Geometry check sheet. Reference: the model listing, model coordinates, mm. Face numbers are marked on the shaded views. A direction names the side the tool comes from. Give positions to 0.01 mm unless a question says otherwise; leave off trailing zeros. Loops run counter-clockwise (first coordinate to the right, second up) from the corner with the lowest first, then second, coordinate; pieces in that order, holes last. Notation, with made-up numbers: (1.5, 29) - (53.5, 29) arc R22 ccw to (53.5, 55) - close; hole circle Ø10 at (72, 31.5). An arc over 180 degrees is marked (long way). One line per question, with ' | ' between items. Start each with the question number.
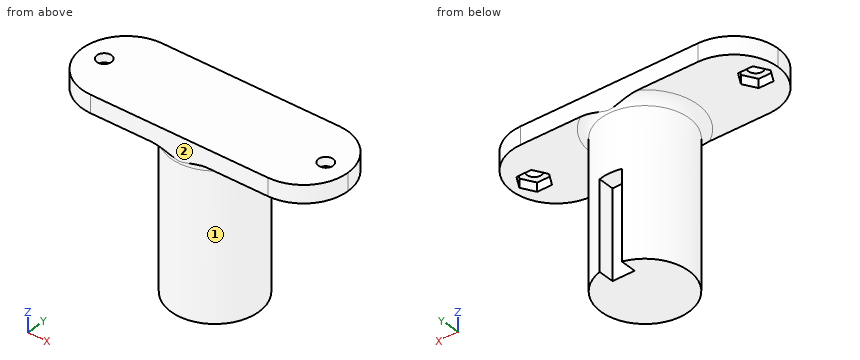
Autodesk Inventor part; units mm, degrees
ref_plane "YZ Plane" through (0, 0, 0) normal (1, 0, 0) x (0, 1, 0)
ref_plane "XZ Plane" through (0, 0, 0) normal (0, 1, 0) x (-1, 0, 0)
ref_plane "XY Plane" through (0, 0, 0) normal (0, 0, 1) x (1, 0, 0)
sketch "Sketch1" plane through (0, 0, 0) normal (0, 0, 1) x (1, 0, 0)
  line L0 (-30, -10) -> (30, -10)
  line L1 (30, -10) -> (30, 10)
  line L2 (30, 10) -> (-30, 10)
  line L3 (-30, 10) -> (-30, -10)
  line L4 (-30, -10) -> (30, 10) construction
  line L5 (30, -10) -> (-30, 10) construction
  circle A0 centre (0, 0) radius 9.9
  circle A1 centre (-25, 0) radius 1.65
  circle A2 centre (25, 0) radius 1.65
  line L6 (-25, 0) -> (25, 0) construction
  point P0 (-30, 0)
  dimension "d0" = 60
  dimension "d1" = 19.8
  dimension "d2" = 20
  dimension "d3" = 50
  dimension "d4" = 3.3
extrude "Extrusion1" add sketch "Sketch1" along normal blind 4 contours L3 L2 L1 L0 | A0
extrude "Extrusion2" add sketch "Sketch1" against normal blind 35 contours A0
fillet "Fillet1" radius 2 1 edges at (-9.9, 0, 0)
fillet "Fillet2" radius 10 4 edges at (30, 10, 2) (30, -10, 2) (-30, 10, 2) (-30, -10, 2)
sketch "Sketch2" plane through (0, 0, -35) normal (0, 0, -1) x (-1, 0, 0)
  circle A0 centre (0, 0) radius 9.9
  line L0 (-2.5, 0) -> (2.5, 0)
  line L1 (2.5, 0) -> (2.5, 12)
  line L2 (2.5, 12) -> (-2.5, 12)
  line L3 (-2.5, 12) -> (-2.5, 0)
  line L4 (-2.5, 6) -> (2.5, 6)
  point P0 (0, 12)
  point P1 (2.5, 9.5791)
  point P2 (-2.5, 9.5791)
  dimension "d11" = 12
  dimension "d12" = 5
  dimension "d13" = 6
extrude "Extrusion3" cut sketch "Sketch2" against normal blind 20 contours L1 L4 L3 A0
sketch "Sketch3" plane through (0, 0, 0) normal (0, 0, -1) x (-1, 0, 0)
  arc A0 (-20, 10) -> (-20, -10) centre (-20, 0) ccw
  line L0 (-6.4506, -10) -> (-20, -10)
  arc A1 (-6.4506, 10) -> (-6.4506, -10) centre (0, 0) ccw
  line L1 (-20, 10) -> (-6.4506, 10)
  circle A2 centre (-25, 0) radius 1.65
  line L2 (-28.3486, 0) -> (-26.6743, 2.9)
  line L3 (-26.6743, 2.9) -> (-23.3257, 2.9)
  line L4 (-23.3257, 2.9) -> (-21.6514, 0)
  line L5 (-21.6514, 0) -> (-23.3257, -2.9)
  line L6 (-23.3257, -2.9) -> (-26.6743, -2.9)
  line L7 (-26.6743, -2.9) -> (-28.3486, 0)
  circle A3 centre (25, 0) radius 1.65
  line L8 (23.3257, 2.9) -> (26.6743, 2.9)
  line L9 (26.6743, 2.9) -> (28.3486, 0)
  line L10 (28.3486, 0) -> (26.6743, -2.9)
  line L11 (26.6743, -2.9) -> (23.3257, -2.9)
  line L12 (23.3257, -2.9) -> (21.6514, 0)
  line L13 (21.6514, 0) -> (23.3257, 2.9)
  point P0 (-25, 2.9)
  dimension "d16" = 5.8
  dimension "d17" = 5.8
extrude "Extrusion4" cut sketch "Sketch3" against normal blind 2 contours L2 L3 L4 L5 L6 L7 | L8 L9 L10 L11 L12 L13
properties part number "GIRO_1" material "Steel, Mild, Welded"
(1) Tool access check on the marked faces 1 and 2. Record the directions out of +Z, -Z, +X, -X, +Y, -Y that give a thin tool (end or side, any length) a straight path to the whole face; none if there is none.
(2) Material ranges on line 1 (X direction, y = 0, z = 3); line 2 (Z direction, x = 10.5, y = 5.25); line 3 (Z direction, x = 22.5, y = 1.25), recorded low to high.
(3) Depth check by flat-ended pin: pin 1 Ø1.7 at (x, y) = (-24.5, -1) entering from -Z; pin 2 Ø1 at (x, z) = (25, 1.5) entering from -Y; pin 3 Ø3 at (y, z) = (0, -11) entering from -X. Enter the tip coordinate at first touch or a pass-through.
(4) Section check B-B, the plane x = 0. Record the boundary of the cut face in (y, z).
(5) Section check D-D, the plane x = 15.5. Record the boundary of the cut face in (y, z).
(6) Section check A-A, the plane x = 24. Record the boundary of the cut face in (y, z).
(7) Section check C-C, the plane z = -19.5. Record the boundary of the cut face in (x, y).
Numbers:
1) face 1: -Z | face 2: +Z, -Z, +X, -X, -Y
2) line 1: -30 to -26.65, -23.35 to 23.35, 26.65 to 30 | line 2: -0.01 to 4 | line 3: 2 to 4
3) pin 1: z = 2 | pin 2: y = -8.93 | pin 3: x = -9.9
4) outline: (-10, -1.38) arc R2 cw to (-9.9, -2) - (-9.9, -35) - (6, -35) - (6, -15) - (9.9, -15) - (9.9, -2) arc R2 cw to (10, -1.38) - (10, 4) - (-10, 4) - close
5) outline: (-10, 0) - (10, 0) - (10, 4) - (-10, 4) - close
6) outline: (-9.17, 0) - (-2.9, 0) - (-2.9, 2) - (-1.31, 2) - (-1.31, 4) - (-9.17, 4) - close; (1.31, 2) - (2.9, 2) - (2.9, 0) - (9.17, 0) - (9.17, 4) - (1.31, 4) - close
7) outline: (-2.5, 6) - (-2.5, 9.58) arc R9.9 ccw (long way) to (2.5, 9.58) - (2.5, 6) - close
